Read the model definition and answer for the solid it produces. Units are mm, in the model's axes. Give positions to 0.01 mm unless a question says otherwise; leave off trailing zeros. Loops run counter-clockwise (first coordinate to the right, second up) from the corner with the lowest first, then second, coordinate; pieces in that order, holes last. Notation, with made-up numbers: (53.5, 1.25) - (64.5, 1.25) arc R33 ccw to (64.5, 36.25) - close; hole circle Ø11 at (29.5, 43.5). An arc over 180 degrees is marked (long way). Write each question's results on one line, items separated by ' | '. Start each with the question number.
Q1. The part is cut by section B-B, the plane z = 2.5. Write down the section's boundary in (x, y), plus the area to 3 significant figures.
Q2. The part is cut by section C-C, the plane x = -4.5. Write down the section's boundary in (y, z), plus the area to 3 significant figures.
Q3. The part is cut by section D-D, the plane y = -7. Write down the section's boundary in (x, z), plus the area to 3 significant figures.
Q4. The part is cut by section A-A, the plane y = 45.5. Write down the section's boundary in (x, z).
Q5. Find the intervals of material crossed by line 1 (Z direction, x = 6, y = 18); line 2 (X direction, y = -22, z = -1.25), in increasing order. Write a range as from..to.
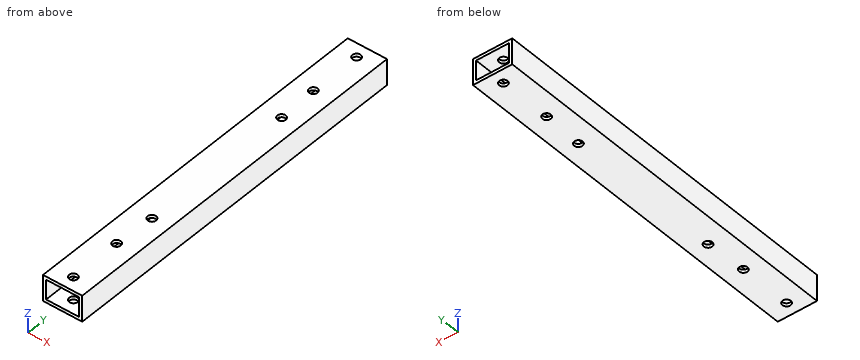
```python
from build123d import *

# Parameters (mm, degrees)
SKETCH_1_W          = 15
SKETCH_1_H          = 10
SKETCH_1_W_2        = 12.6
SKETCH_1_H_2        = 7.6
EXTRUDE_1_DEPTH     = 70.5
SKETCH_2_R          = 1.6
CUT_EXTRUDE_1_DEPTH = 100
SKETCH_3_R          = 1.6
CUT_EXTRUDE_2_DEPTH = 10


with BuildPart() as part:
    # ｽｹｯﾁ1 → ﾎﾞｽ - 押し出し1 (new, symmetric)
    with BuildSketch(Plane(origin=(0, 0, 0), x_dir=(1, 0, 0), z_dir=(0, 1, 0))):
        Rectangle(SKETCH_1_W, SKETCH_1_H)
        Rectangle(SKETCH_1_W_2, SKETCH_1_H_2, mode=Mode.SUBTRACT)
    extrude(amount=EXTRUDE_1_DEPTH, both=True)

    # ｽｹｯﾁ2 → ｶｯﾄ - 押し出し1 (cut)
    with BuildSketch(Plane(origin=(0, 0, -5), x_dir=(-1, 0, 0), z_dir=(0, 0, -1))):
        with Locations((0, -65.5)):
            Circle(SKETCH_2_R)
        with Locations((0, -45.5)):
            Circle(SKETCH_2_R)
        with Locations(Location((0, 45.5, 0), (0, 0, 180))):
            Circle(SKETCH_2_R)
        with Locations(Location((0, 65.5, 0), (0, 0, 180))):
            Circle(SKETCH_2_R)
    extrude(amount=-CUT_EXTRUDE_1_DEPTH, mode=Mode.SUBTRACT)

    # ｽｹｯﾁ3 → ｶｯﾄ - 押し出し2 (cut)
    with BuildSketch(Plane(origin=(0, 0, -5), x_dir=(-1, 0, 0), z_dir=(0, 0, -1))):
        with Locations((-0.676513704, -30)):
            Circle(SKETCH_3_R)
        with Locations((-0.676513704, 30)):
            Circle(SKETCH_3_R)
    extrude(amount=-CUT_EXTRUDE_2_DEPTH, mode=Mode.SUBTRACT)


solid = part.part
```
Check sheet entries:
1) outline: (-7.5, -70.5) - (-6.3, -70.5) - (-6.3, 70.5) - (-7.5, 70.5) - close; (6.3, -70.5) - (7.5, -70.5) - (7.5, 70.5) - (6.3, 70.5) - close | area: 338 mm^2
2) outline: (-70.5, -5) - (70.5, -5) - (70.5, -3.8) - (-70.5, -3.8) - close; (-70.5, 3.8) - (70.5, 3.8) - (70.5, 5) - (-70.5, 5) - close | area: 338 mm^2
3) outline: (-7.5, -5) - (7.5, -5) - (7.5, 5) - (-7.5, 5) - close; hole (-6.3, -3.8) - (6.3, -3.8) - (6.3, 3.8) - (-6.3, 3.8) - close | area: 54.2 mm^2
4) outline: (-7.5, -5) - (-1.6, -5) - (-1.6, -3.8) - (-6.3, -3.8) - (-6.3, 3.8) - (-1.6, 3.8) - (-1.6, 5) - (-7.5, 5) - close; (1.6, -5) - (7.5, -5) - (7.5, 5) - (1.6, 5) - (1.6, 3.8) - (6.3, 3.8) - (6.3, -3.8) - (1.6, -3.8) - close
5) line 1: z = -5..-3.8, 3.8..5 | line 2: x = -7.5..-6.3, 6.3..7.5
